```python
from build123d import *

# Parameters (mm, degrees)
SKETCH1_W           = 118
SKETCH1_H           = 47
BOSS_EXTRUDE1_DEPTH = 5
FILLET1_R           = 6
SKETCH4_R           = 2.25
CUT_EXTRUDE1_DEPTH  = 64.704395453
CUT_EXTRUDE2_DEPTH  = 2.5
CUT_EXTRUDE3_DEPTH  = 3
FILLET2_R           = 1
SKETCH7_W           = 4
SKETCH7_H           = 1
CUT_EXTRUDE4_DEPTH  = 1.5
FILLET3_START       = 3.5
FILLET3_DEPTH       = 2.5
FILLET3_2_DEPTH     = 1.5
SKETCH8_R           = 1.5
CUT_EXTRUDE5_DEPTH  = 64.578691399


with BuildPart() as part:
    # Sketch1 → Boss-Extrude1 (new body)
    with BuildSketch(Plane(origin=(0, 0, 0), x_dir=(1, 0, 0), z_dir=(0, 1, 0))):
        Rectangle(SKETCH1_W, SKETCH1_H)
    extrude(amount=BOSS_EXTRUDE1_DEPTH)

    # Fillet1
    fillet1_edges = [part.edges().sort_by_distance(p)[0] for p in [
        (59, 2.5, 23.5),
        (-59, 2.5, 23.5),
        (-59, 2.5, -23.5),
        (59, 2.5, -23.5),
    ]]
    fillet(fillet1_edges, radius=FILLET1_R)

    # Sketch4 → Cut-Extrude1 (cut, through all)
    with BuildSketch(Plane(origin=(0, 5, 0), x_dir=(1, 0, 0), z_dir=(0, 1, 0))):
        with Locations(Location((53, -17.5, 0), (0, 0, 270))):
            Circle(SKETCH4_R)
        with Locations(Location((-53, -17.5, 0), (0, 0, 90))):
            Circle(SKETCH4_R)
        with Locations(Location((53, 17.5, 0), (0, 0, 90))):
            Circle(SKETCH4_R)
        with Locations(Location((-53, 17.5, 0), (0, 0, 270))):
            Circle(SKETCH4_R)
    extrude(amount=-CUT_EXTRUDE1_DEPTH, mode=Mode.SUBTRACT)

    # Sketch5 → Cut-Extrude2 (cut)
    with BuildSketch(Plane.XZ):
        Polygon((50.907105274, -13.875), (48.814210548, -17.5), (50.907105274, -21.125), (55.092894726, -21.125), (57.185789452, -17.5), (55.092894726, -13.875), align=None)
        Polygon((57.185789452, 17.5), (55.092894726, 13.875), (50.907105274, 13.875), (48.814210548, 17.5), (50.907105274, 21.125), (55.092894726, 21.125), align=None)
        Polygon((-57.185789452, -17.5), (-55.092894726, -13.875), (-50.907105274, -13.875), (-48.814210548, -17.5), (-50.907105274, -21.125), (-55.092894726, -21.125), align=None)
        Polygon((-55.092894726, 13.875), (-50.907105274, 13.875), (-48.814210548, 17.5), (-50.907105274, 21.125), (-55.092894726, 21.125), (-57.185789452, 17.5), align=None)
    extrude(amount=-CUT_EXTRUDE2_DEPTH, mode=Mode.SUBTRACT)

    # Sketch6 → Cut-Extrude3 (cut)
    with BuildSketch(Plane(origin=(0, 5, 0), x_dir=(1, 0, 0), z_dir=(0, 1, 0))):
        with BuildLine():
            Line((57, 13.027864045), (57, -13.027864045))
            ThreePointArc((57, -13.027864045), (48.757359313, -13.257359313), (48.527864045, -21.5))
            Line((48.527864045, -21.5), (-48.527864045, -21.5))
            ThreePointArc((-48.527864045, -21.5), (-48.757359313, -13.257359313), (-57, -13.027864045))
            Line((-57, -13.027864045), (-57, 13.027864045))
            ThreePointArc((-57, 13.027864045), (-48.757359313, 13.257359313), (-48.527864045, 21.5))
            Line((-48.527864045, 21.5), (48.527864045, 21.5))
            ThreePointArc((48.527864045, 21.5), (48.757359313, 13.257359313), (57, 13.027864045))
        make_face()
    extrude(amount=-CUT_EXTRUDE3_DEPTH, mode=Mode.SUBTRACT)

    # Fillet2
    fillet2_edges = [part.edges().sort_by_distance(p)[0] for p in [
        (48.527864045, 3.5, -21.5),
        (57, 3.5, -13.027864045),
        (57, 3.5, 13.027864045),
        (48.527864045, 3.5, 21.5),
        (-48.527864045, 3.5, 21.5),
        (-57, 3.5, 13.027864045),
        (-57, 3.5, -13.027864045),
        (-48.527864045, 3.5, -21.5),
    ]]
    fillet(fillet2_edges, radius=FILLET2_R)

    # Sketch7 → Cut-Extrude4 (cut)
    with BuildSketch(Plane(origin=(0, 5, 0), x_dir=(1, 0, 0), z_dir=(0, 1, 0))):
        with BuildLine():
            Line((-48, -21.5), (-48, -22.5))
            Line((-48, -22.5), (-38, -22.5))
            Line((-38, -22.5), (-38, -21.5))
            Line((-38, -21.5), (-46.67544468, -21.5))
            ThreePointArc((-46.67544468, -21.5), (-47.520598934, -21.034522484), (-47.578952583, -20.071428571))
            ThreePointArc((-47.578952583, -20.071428571), (-47.640934848, -20.198225473), (-47.705882353, -20.323529412))
            ThreePointArc((-47.705882353, -20.323529412), (-47.92535625, -20.893660937), (-48, -21.5))
        make_face()
        with Locations((-42, 22)):
            Rectangle(SKETCH7_W, SKETCH7_H)
        with Locations((-30, 22)):
            Rectangle(SKETCH7_W, SKETCH7_H)
        with Locations((-18, 22)):
            Rectangle(SKETCH7_W, SKETCH7_H)
        with Locations((-6, 22)):
            Rectangle(SKETCH7_W, SKETCH7_H)
        with Locations((6, 22)):
            Rectangle(SKETCH7_W, SKETCH7_H)
        with Locations((18, 22)):
            Rectangle(SKETCH7_W, SKETCH7_H)
        with Locations((30, 22)):
            Rectangle(SKETCH7_W, SKETCH7_H)
        with Locations((42, 22)):
            Rectangle(SKETCH7_W, SKETCH7_H)
    extrude(amount=-CUT_EXTRUDE4_DEPTH, mode=Mode.SUBTRACT)

    # Fillet3: read off the stored shape, not the designer's step
    # Fillet3 outline → Fillet3 (cut)
    with BuildSketch(Plane(origin=(0, 0, 0), x_dir=(1, 0, 0), z_dir=(0, 1, 0)).offset(FILLET3_START)):
        with BuildLine():
            Line((-40, 21.5), (-39.5, 21.5))
            ThreePointArc((-39.5, 21.5), (-39.853553391, 21.646446609), (-40, 22))
            Line((-40, 22), (-40, 21.5))
        make_face()
        with BuildLine():
            Line((-28, 21.5), (-27.5, 21.5))
            ThreePointArc((-27.5, 21.5), (-27.853553391, 21.646446609), (-28, 22))
            Line((-28, 22), (-28, 21.5))
        make_face()
        with BuildLine():
            Line((-16, 21.5), (-15.5, 21.5))
            ThreePointArc((-15.5, 21.5), (-15.853553391, 21.646446609), (-16, 22))
            Line((-16, 22), (-16, 21.5))
        make_face()
        with BuildLine():
            Line((-4, 21.5), (-3.5, 21.5))
            ThreePointArc((-3.5, 21.5), (-3.853553391, 21.646446609), (-4, 22))
            Line((-4, 22), (-4, 21.5))
        make_face()
        with BuildLine():
            Line((8, 21.5), (8.5, 21.5))
            ThreePointArc((8.5, 21.5), (8.146446609, 21.646446609), (8, 22))
            Line((8, 22), (8, 21.5))
        make_face()
        with BuildLine():
            Line((20, 21.5), (20.5, 21.5))
            ThreePointArc((20.5, 21.5), (20.146446609, 21.646446609), (20, 22))
            Line((20, 22), (20, 21.5))
        make_face()
        with BuildLine():
            Line((32, 21.5), (32.5, 21.5))
            ThreePointArc((32.5, 21.5), (32.146446609, 21.646446609), (32, 22))
            Line((32, 22), (32, 21.5))
        make_face()
        with BuildLine():
            ThreePointArc((44.5, 21.5), (44.146446609, 21.646446609), (44, 22))
            Line((44, 22), (44, 21.5))
            Line((44, 21.5), (44.5, 21.5))
        make_face()
        with BuildLine():
            Line((39.5, 21.5), (40, 21.5))
            Line((40, 21.5), (40, 22))
            ThreePointArc((40, 22), (39.853553391, 21.646446609), (39.5, 21.5))
        make_face()
        with BuildLine():
            Line((27.5, 21.5), (28, 21.5))
            Line((28, 21.5), (28, 22))
            ThreePointArc((28, 22), (27.853553391, 21.646446609), (27.5, 21.5))
        make_face()
        with BuildLine():
            Line((15.5, 21.5), (16, 21.5))
            Line((16, 21.5), (16, 22))
            ThreePointArc((16, 22), (15.853553391, 21.646446609), (15.5, 21.5))
        make_face()
        with BuildLine():
            Line((3.5, 21.5), (4, 21.5))
            Line((4, 21.5), (4, 22))
            ThreePointArc((4, 22), (3.853553391, 21.646446609), (3.5, 21.5))
        make_face()
        with BuildLine():
            Line((-8.5, 21.5), (-8, 21.5))
            Line((-8, 21.5), (-8, 22))
            ThreePointArc((-8, 22), (-8.146446609, 21.646446609), (-8.5, 21.5))
        make_face()
        with BuildLine():
            Line((-20.5, 21.5), (-20, 21.5))
            Line((-20, 21.5), (-20, 22))
            ThreePointArc((-20, 22), (-20.146446609, 21.646446609), (-20.5, 21.5))
        make_face()
        with BuildLine():
            Line((-32.5, 21.5), (-32, 21.5))
            Line((-32, 21.5), (-32, 22))
            ThreePointArc((-32, 22), (-32.146446609, 21.646446609), (-32.5, 21.5))
        make_face()
        with BuildLine():
            Line((-44.5, 21.5), (-44, 21.5))
            Line((-44, 21.5), (-44, 22))
            ThreePointArc((-44, 22), (-44.146446609, 21.646446609), (-44.5, 21.5))
        make_face()
        with BuildLine():
            Line((-38, -21.5), (-38, -22))
            ThreePointArc((-38, -22), (-37.853553391, -21.646446609), (-37.5, -21.5))
            Line((-37.5, -21.5), (-38, -21.5))
        make_face()
    extrude(amount=FILLET3_DEPTH, mode=Mode.SUBTRACT)

    # Fillet3 2 outline → Fillet3 2 (add)
    with BuildSketch(Plane(origin=(0, 0, 0), x_dir=(1, 0, 0), z_dir=(0, 1, 0)).offset(FILLET3_START)):
        with BuildLine():
            ThreePointArc((43.5, 22.5), (43.853553391, 22.353553391), (44, 22))
            Line((44, 22), (44, 22.5))
            Line((44, 22.5), (43.5, 22.5))
        make_face()
        with BuildLine():
            ThreePointArc((40, 22), (40.146446609, 22.353553391), (40.5, 22.5))
            Line((40.5, 22.5), (40, 22.5))
            Line((40, 22.5), (40, 22))
        make_face()
        with BuildLine():
            ThreePointArc((31.5, 22.5), (31.853553391, 22.353553391), (32, 22))
            Line((32, 22), (32, 22.5))
            Line((32, 22.5), (31.5, 22.5))
        make_face()
        with BuildLine():
            ThreePointArc((28, 22), (28.146446609, 22.353553391), (28.5, 22.5))
            Line((28.5, 22.5), (28, 22.5))
            Line((28, 22.5), (28, 22))
        make_face()
        with BuildLine():
            ThreePointArc((16, 22), (16.146446609, 22.353553391), (16.5, 22.5))
            Line((16.5, 22.5), (16, 22.5))
            Line((16, 22.5), (16, 22))
        make_face()
        with BuildLine():
            ThreePointArc((7.5, 22.5), (7.853553391, 22.353553391), (8, 22))
            Line((8, 22), (8, 22.5))
            Line((8, 22.5), (7.5, 22.5))
        make_face()
        with BuildLine():
            ThreePointArc((4, 22), (4.146446609, 22.353553391), (4.5, 22.5))
            Line((4.5, 22.5), (4, 22.5))
            Line((4, 22.5), (4, 22))
        make_face()
        with BuildLine():
            ThreePointArc((-4.5, 22.5), (-4.146446609, 22.353553391), (-4, 22))
            Line((-4, 22), (-4, 22.5))
            Line((-4, 22.5), (-4.5, 22.5))
        make_face()
        with BuildLine():
            ThreePointArc((-8, 22), (-7.853553391, 22.353553391), (-7.5, 22.5))
            Line((-7.5, 22.5), (-8, 22.5))
            Line((-8, 22.5), (-8, 22))
        make_face()
        with BuildLine():
            ThreePointArc((-16.5, 22.5), (-16.146446609, 22.353553391), (-16, 22))
            Line((-16, 22), (-16, 22.5))
            Line((-16, 22.5), (-16.5, 22.5))
        make_face()
        with BuildLine():
            ThreePointArc((-20, 22), (-19.853553391, 22.353553391), (-19.5, 22.5))
            Line((-19.5, 22.5), (-20, 22.5))
            Line((-20, 22.5), (-20, 22))
        make_face()
        with BuildLine():
            ThreePointArc((-28.5, 22.5), (-28.146446609, 22.353553391), (-28, 22))
            Line((-28, 22), (-28, 22.5))
            Line((-28, 22.5), (-28.5, 22.5))
        make_face()
        with BuildLine():
            ThreePointArc((-32, 22), (-31.853553391, 22.353553391), (-31.5, 22.5))
            Line((-31.5, 22.5), (-32, 22.5))
            Line((-32, 22.5), (-32, 22))
        make_face()
        with BuildLine():
            ThreePointArc((-40.5, 22.5), (-40.146446609, 22.353553391), (-40, 22))
            Line((-40, 22), (-40, 22.5))
            Line((-40, 22.5), (-40.5, 22.5))
        make_face()
        with BuildLine():
            ThreePointArc((-44, 22), (-43.853553391, 22.353553391), (-43.5, 22.5))
            Line((-43.5, 22.5), (-44, 22.5))
            Line((-44, 22.5), (-44, 22))
        make_face()
        with BuildLine():
            Line((-48, -22.5), (-47.5, -22.5))
            ThreePointArc((-47.5, -22.5), (-47.853553391, -22.353553391), (-48, -22))
            Line((-48, -22), (-48, -22.5))
        make_face()
        with BuildLine():
            ThreePointArc((-38, -22), (-38.146446609, -22.353553391), (-38.5, -22.5))
            Line((-38.5, -22.5), (-38, -22.5))
            Line((-38, -22.5), (-38, -22))
        make_face()
    extrude(amount=FILLET3_2_DEPTH)

    # Sketch8 → Cut-Extrude5 (cut, through all)
    with BuildSketch(Plane(origin=(0, 2, 0), x_dir=(1, 0, 0), z_dir=(0, 1, 0))):
        with Locations(Location((-52.5, 0, 0), (0, 0, 270))):
            Circle(SKETCH8_R)
        with Locations(Location((52.5, 0, 0), (0, 0, 90))):
            Circle(SKETCH8_R)
    extrude(amount=-CUT_EXTRUDE5_DEPTH, mode=Mode.SUBTRACT)


solid = part.part
```
Geometry check sheet. Reference: the model listing, model coordinates, mm. A direction names the side the tool comes from. Coordinates: 2 decimals unless noted, no trailing zeros. Loops run counter-clockwise (first coordinate to the right, second up) from the corner with the lowest first, then second, coordinate; pieces in that order, holes last.
Item 1: Access from +Z, -Z, +X, -X, +Y, -Y to the whole of each face (thin tool, end or side, straight path). Record for faces 1 (the face through (-1, 0, 0)), 2 (the face through (-48.831, 3.521, -13.185)), 3 (the face through (53, 1, 21.125)).
Item 2: Sectioned sample at C-C, the plane x = 34. Record the boundary of the cut face in (y, z).
Item 3: Go/stop test with flat-tipped pins: pin 1 Ø0.8 at (x, z) = (42, -22) entering from +Y; pin 2 Ø5 at (x, z) = (21.5, 2) entering from +Y. Record where each tip stops, or that it passes through.
Item 4: Sectioned sample at A-A, the plane z = 0. Record the boundary of the cut face in (x, y).
Item 5: Thickness scan on line 1 (X direction, y = 1, z = -17.5); line 2 (X direction, y = 3.9, z = -17.5); line 3 (Z direction, x = 13, y = 3.4). Record the ranges inside material, lowest first.
Item 6: Sectioned sample at D-D, the plane z = 5. Record the boundary of the cut face in (x, y).
Item 7: Sectioned sample at B-B, the plane y = 1.25. Count the separate pieces of the cut face and the enclosed holes in it, then the cut area to 3 significant figures.
Check result:
1. face 1: +Z, -Z, +X, -X, -Y
1. face 2: +Y
1. face 3: -Y
2. outline: (0, -23.5) - (5, -23.5) - (5, -21.5) - (2, -21.5) - (2, 21.5) - (5, 21.5) - (5, 23.5) - (0, 23.5) - close
3. pin 1: stops at y = 3.5
3. pin 2: stops at y = 2
4. outline: (-59, 0) - (-54, 0) - (-54, 2) - (-57, 2) - (-57, 5) - (-59, 5) - close; (-51, 0) - (51, 0) - (51, 2) - (-51, 2) - close; (54, 0) - (59, 0) - (59, 5) - (57, 5) - (57, 2) - (54, 2) - close
5. line 1: x = -59 to -57.19, -48.81 to 48.81, 57.19 to 59
5. line 2: x = -59 to -55.25, -50.75 to -47, 47 to 50.75, 55.25 to 59
5. line 3: z = -23.5 to -21.5, 21.5 to 23.5
6. outline: (-59, 0) - (59, 0) - (59, 5) - (57, 5) - (57, 2) - (-57, 2) - (-57, 5) - (-59, 5) - close
7. separate pieces: 1
7. enclosed holes: 6
7. area: 5,320 mm2
